Design review of the part built by this model. Coordinates are the model's own, in mm. Give positions to 0.01 mm unless a question says otherwise; leave off trailing zeros. Write each loop counter-clockwise with the first axis right and the second up, starting at its lowest first coordinate (ties: lowest second). Pieces come first, ordered by that corner, then holes. Notation, with made-up numbers: (59, 47.5) -> (96, 47.5) arc R14 cw to (96, 73.5) -> close; hole circle Ø11 at (-6, 8). An arc over 180 degrees is marked (long way). Write each question's results on one line, items separated by ' | '. Start each with the question number.
(1) To check wall thickness, follow probe 1 along Y at (x, z) = (0, -4.5) (1 decimal); probe 2 along Y at (x, z) = (2, -1.25); probe 3 along X at (y, z) = (10, -7). State the ranges of each line that lie inside material, in increasing order.
(2) Take a section at A-A (x = 0). State the section outline as (y, z) points (1 decimal), plus the area to 3 significant figures.
(3) Clearance check with flat-ended pins moving along their axes: pin 1 (3 mm diameter, centred on x = -7.5, y = 9, fed in from +Z); pin 2 (5.5 mm diameter, centred on x = 0, y = 0, fed in from +Z); pin 3 (1 mm diameter, centred on x = -4.5, z = -8, fed in from -Y); pin 4 (1.5 mm diameter, centred on y = -6.5, z = -4, fed in from -X). State where each tip first meets the part, or that it passes through.
(4) Take a section at B-B (z = -1). State the section outline as (x, y) points (1 decimal).
(5) Take a section at C-C (z = -7.5). State the section outline as (x, y) points (1 decimal), plus the area to 3 significant figures.
(6) Mouldability with a two-part tool opening along Y and no side actions: class faces 1 (the face through (-0.35, -15.87, -4.73)), 2 (the face through (-3.78, -2.9, -4.7)), 3 (the face through (0.068, 15.875, -4.731)) as released by +Y, released by -Y, zero draft, split by the parting line, or undercut.
from build123d import *

# Parameters (mm, degrees)
SKETCH1_R           = 15.875
SKETCH1_R_2         = 4.7625
SKETCH1_R_3         = 2.3749
BOSS_EXTRUDE1_DEPTH = 9.525
CUT_EXTRUDE1_DEPTH  = 10.525
FILLET1_R           = 2.54
FILLET2_R           = 2.54


with BuildPart() as part:
    # Sketch1 → Boss-Extrude1 (new body)
    with BuildSketch(Plane.XY):
        Circle(SKETCH1_R)
        Circle(SKETCH1_R_2, mode=Mode.SUBTRACT)
        with Locations((0, 9.525)):
            Circle(SKETCH1_R_3, mode=Mode.SUBTRACT)
    extrude(amount=-BOSS_EXTRUDE1_DEPTH)

    # Sketch2 → Cut-Extrude1 (cut, through all)
    with BuildSketch(Plane.XY):
        with BuildLine():
            ThreePointArc((-15.875, 0), (-8.06886604, 5.915724645), (-4.7752, 15.139785004))
            ThreePointArc((-4.7752, 15.139785004), (-12.802771673, 9.386408392), (-15.875, 0))
        make_face()
        with BuildLine():
            ThreePointArc((15.875, 0), (8.06886604, 5.915724645), (4.7752, 15.139785004))
            ThreePointArc((4.7752, 15.139785004), (12.802771673, 9.386408392), (15.875, 0))
        make_face()
    extrude(amount=-CUT_EXTRUDE1_DEPTH, mode=Mode.SUBTRACT)

    # Fillet1
    fillet1_edges = [part.edges().sort_by_distance(p)[0] for p in [
        (0, 15.875, 0),
        (0, -15.875, 0),
        (-8.06886604, 5.915724645, 0),
        (8.06886604, 5.915724645, 0),
    ]]
    fillet(fillet1_edges, radius=FILLET1_R)

    # Fillet2
    fillet2_edges = [part.edges().sort_by_distance(p)[0] for p in [
        (0, 15.875, -9.525),
        (0, -15.875, -9.525),
        (-8.06886604, 5.915724645, -9.525),
        (8.06886604, 5.915724645, -9.525),
    ]]
    fillet(fillet2_edges, radius=FILLET2_R)


solid = part.part
Report:
1) probe 1: -15.9 to -4.8, 4.8 to 7.2, 11.9 to 15.9 | probe 2: -15.39 to -4.32, 4.32 to 8.24, 10.81 to 15.39 | probe 3: -5.85 to -2.33, 2.33 to 5.85
2) outline: (-15.9, -7) arc R2.5 ccw to (-13.3, -9.5) -> (-4.8, -9.5) -> (-4.8, 0) -> (-13.3, 0) arc R2.5 ccw to (-15.9, -2.5) -> close; (4.8, -9.5) -> (7.2, -9.5) -> (7.2, 0) -> (4.8, 0) -> close; (11.9, -9.5) -> (13.3, -9.5) arc R2.5 ccw to (15.9, -7) -> (15.9, -2.5) arc R2.5 ccw to (13.3, 0) -> (11.9, 0) -> close | area: 161 mm2
3) pin 1: z = -1.19 | pin 2: through | pin 3: y = -15.23 | pin 4: x = -14.8
4) outline: (-15.4, -0.4) arc R15.4 ccw to (15.4, -0.4) arc R17.7 cw to (4.3, 14.7) arc R15.4 ccw to (-4.3, 14.7) arc R17.7 cw to start; hole circle Ø9.5 at (0, 0); hole circle Ø4.7 at (0, 9.5)
5) outline: (-15.8, 0) arc R15.8 ccw to (15.8, 0) arc R17.2 cw to (4.7, 15.1) arc R15.8 ccw to (-4.7, 15.1) arc R17.2 cw to start; hole circle Ø9.5 at (0, 0); hole circle Ø4.7 at (0, 9.5) | area: 548 mm2
6) face 1: released by -Y | face 2: undercut | face 3: released by +Y
